The listing builds one solid part. Answer for the finished solid, in the listing's coordinates (mm). A direction names the side the tool comes from. Give positions to 0.01 mm unless a question says otherwise; leave off trailing zeros. Loops run counter-clockwise (first coordinate to the right, second up) from the corner with the lowest first, then second, coordinate; pieces in that order, holes last. Notation, with made-up numbers: (5, 8) - (48, 8) arc R10 ccw to (48, 16) - close; hole circle Ø3 at (67.25, -18). An arc over 180 degrees is marked (long way). Answer as CSV lines item,"result". Start each with the question number.
1) Find the intervals of material crossed by line 1 along X through (y, z) = (4.15, 0); line 2 along X through (y, z) = (0.9, 0); line 3 along Y through (x, z) = (-17, 16.5), in increasing order.
2) A cutting plane is placed at D-D (x = 31.75). Determine the outline of the cut face in (y, z) (3 decimals).
3) A cutting plane is placed at B-B (z = -21.59). Determine the outline of the cut face in (x, y).
4) For faces 1 (the face through (-12.677, 1.252, -15.098)), 2 (the face through (-8, 0, 8)), 3 (the face through (32.5, 2.54, -2.2)), determine the directions among +Z, -Z, +X, -X, +Y, -Y from which every point of the face is accessible in a straight line to the end or side of a thin tool.
5) A cutting plane is placed at C-C (y = 3.5). Give the number of separate pieces and of enclosed holes in the cut face, and give its area (3 significant figures).
6) Flat-ended cylindrical pins translate along their axes: pin 1 (3.5 mm diameter, centred on x = -1, z = -23, fed in from +Y); pin 2 (2 mm diameter, centred on x = 15.5, z = -17.5, fed in from +Y); pin 3 (5 mm diameter, centred on x = 12, y = 3, fed in from -Z); pin 4 (8 mm diameter, centred on x = 31.75, z = 0, fed in from -Y). Find the tip coordinate at first contact, or state that the pin passes through.
7) For a pull along Z with two mould halves and no side action, classify faces 4 (the face through (-23.183, 3.131, -30.235)), 5 (the face through (1, 6.35, -1)), 6 (the face through (0, 5.08, 0)) as pulls with the +Z half, pulls with the -Z half, needs draft (parallel to the pull), parting line crosses it, or undercut.
```python
from build123d import *

# Parameters (mm, degrees)
SKETCH1_R               = 38.1
BOSS_EXTRUDE1_DEPTH     = 6.35
CUT_EXTRUDE1_DEPTH      = 55.254423783
CUT_EXTRUDE1_DEPTH_BACK = 3.81
SKETCH2_R               = 3.429
CUT_EXTRUDE2_DEPTH      = 55.254423783
CUT_EXTRUDE2_DEPTH_BACK = 55.254423783
SKETCH2_3_R             = 2.159
SKETCH4_R               = 6.910573657
BOSS_EXTRUDE2_DEPTH     = 1.27
BOSS_EXTRUDE3_START     = 3.81
SKETCH5_R               = 6.35
BOSS_EXTRUDE3_DEPTH     = 3.81
FILLET1_R               = 3.81
FILLET2_R               = 0.635


with BuildPart() as part:
    # Sketch1 → Boss-Extrude1 (new body)
    with BuildSketch(Plane(origin=(0, 0, 0), x_dir=(1, 0, 0), z_dir=(0, 1, 0))):
        with Locations(Location((0, 0, 0), (0, 0, 270))):
            Circle(SKETCH1_R)
        with BuildLine():
            Line((-1.786407019, 2.487499957), (1.786407019, 2.487499957))
            ThreePointArc((1.786407019, 2.487499957), (0, -3.062499971), (-1.786407019, 2.487499957))
        make_face(mode=Mode.SUBTRACT)
    extrude(amount=BOSS_EXTRUDE1_DEPTH)

    # Sketch2 → Cut-Extrude1 (cut, two sides: drawn at the far end of the back side and taken through both)
    with BuildSketch(Plane(origin=(0, 6.35, 0), x_dir=(1, 0, 0), z_dir=(0, 1, 0)).offset(-CUT_EXTRUDE1_DEPTH_BACK)):
        with Locations(Location((-20.32, 0, 0), (0, 0, 90))):
            Circle(SKETCH2_R)
        with Locations(Location((-14.8174226, 14.8174226, 0), (0, 0, 90))):
            Circle(SKETCH2_R)
        with Locations(Location((0, 21.59, 0), (0, 0, 90))):
            Circle(SKETCH2_R)
        with Locations(Location((16.164461018, 16.164461018, 0), (0, 0, 90))):
            Circle(SKETCH2_R)
        with Locations(Location((31.75, 0, 0), (0, 0, 90))):
            Circle(SKETCH2_R)
    extrude(amount=CUT_EXTRUDE1_DEPTH + CUT_EXTRUDE1_DEPTH_BACK, mode=Mode.SUBTRACT)

    # Sketch2<3> → Cut-Extrude2 (cut, two sides: drawn at the far end of the back side and taken through both)
    with BuildSketch(Plane(origin=(0, 6.35, 0), x_dir=(1, 0, 0), z_dir=(0, 1, 0)).offset(-CUT_EXTRUDE2_DEPTH_BACK)):
        with Locations(Location((-20.32, 0, 0), (0, 0, 270))):
            Circle(SKETCH2_3_R)
        with Locations(Location((-14.8174226, 14.8174226, 0), (0, 0, 270))):
            Circle(SKETCH2_3_R)
        with Locations(Location((0, 21.59, 0), (0, 0, 270))):
            Circle(SKETCH2_3_R)
        with Locations(Location((16.164461018, 16.164461018, 0), (0, 0, 270))):
            Circle(SKETCH2_3_R)
        with Locations(Location((31.75, 0, 0), (0, 0, 270))):
            Circle(SKETCH2_3_R)
    extrude(amount=CUT_EXTRUDE2_DEPTH + CUT_EXTRUDE2_DEPTH_BACK, mode=Mode.SUBTRACT)

    # Sketch4 → Boss-Extrude2 (add)
    with BuildSketch(Plane(origin=(0, 6.35, 0), x_dir=(1, 0, 0), z_dir=(0, 1, 0))):
        Circle(SKETCH4_R)
    extrude(amount=-BOSS_EXTRUDE2_DEPTH)

    # Sketch5 → Boss-Extrude3 (add)
    with BuildSketch(Plane.XZ.offset(BOSS_EXTRUDE3_START)):
        with Locations(Location((0, 0, 0), (0, 0, 90))):
            Circle(SKETCH5_R)
        with BuildLine():
            Line((-1.786407019, -2.487499957), (1.786407019, -2.487499957))
            ThreePointArc((1.786407019, -2.487499957), (0, 3.062499971), (-1.786407019, -2.487499957))
        make_face(mode=Mode.SUBTRACT)
    extrude(amount=-BOSS_EXTRUDE3_DEPTH)

    # Fillet1
    fillet1_edges = [part.edges().sort_by_distance(p)[0] for p in [
        (0, 0, -6.35),
    ]]
    fillet(fillet1_edges, radius=FILLET1_R - 0.0001)  # a hair under: the kernel refuses the full size

    # Fillet2
    fillet2_edges = [part.edges().sort_by_distance(p)[0] for p in [
        (31.75, 6.35, 3.429),
    ]]
    fillet(fillet2_edges, radius=FILLET2_R)


solid = part.part
```
Ans:
1,line 1,"-38.1 to -23.75, -16.89 to -3.06, 3.06 to 28.32, 35.18 to 38.1"
1,line 2,"-38.1 to -22.48, -18.16 to -3.06, 3.06 to 29.59, 33.91 to 38.1"
1,line 3,"0 to 6.35"
2,outline,"(0, -21.061) - (6.35, -21.061) - (6.35, -4.064) arc R0.635 ccw to (5.715, -3.429) - (2.54, -3.429) - (2.54, -2.159) - (0, -2.159) - close; (0, 2.159) - (2.54, 2.159) - (2.54, 3.429) - (5.715, 3.429) arc R0.635 ccw to (6.35, 4.064) - (6.35, 21.061) - (0, 21.061) - close"
3,outline,"(-31.39, 0) - (-2.16, 0) - (-2.16, 2.54) - (-3.43, 2.54) - (-3.43, 6.35) - (-31.39, 6.35) - close; (2.16, 0) - (31.39, 0) - (31.39, 6.35) - (3.43, 6.35) - (3.43, 2.54) - (2.16, 2.54) - close"
4,face 1,"+Y, -Y"
4,face 2,"-Y"
4,face 3,"+Y"
5,separate pieces,"1"
5,enclosed holes,"6"
5,area,"4,350 mm2"
6,pin 1,"y = 6.35"
6,pin 2,"y = 2.54"
6,pin 3,"z = -36.9"
6,pin 4,"y = 0"
7,face 4,"parting line crosses it"
7,face 5,"needs draft"
7,face 6,"undercut"
